Answer from the drawing. Dimensions are ordinates in mm from the lowest x, y and z of the part. Give positions to 0.01 mm unless a question says otherwise; leave off trailing zeros. Order: outer loops, then holes, each group sorted by start corner. A loop starts at its lowest first (then second) coordinate and runs counter-clockwise, first axis right, second up. Notation, with made-up numbers: M -31.75,-11 L -7.75,-11 A10 ccw -7.75,-7 Z; hole C 39,44.25 d5. An arc over 180 degrees is marked long. One line per item, written item: value.
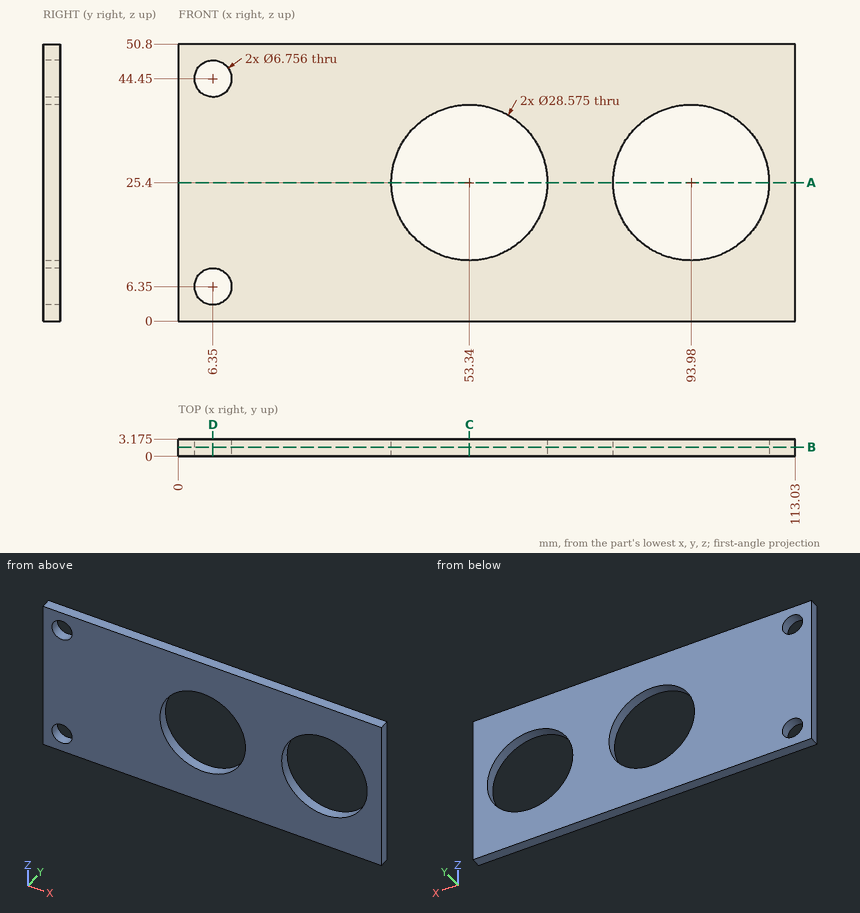
(1) Section C-C, the plane x = 53.34 is taken. Give the vertices of the cut face in (y, z) (1 decimal).
Findings:
outline: M 0,0 L 3.2,0 L 3.2,11.1 L 0,11.1 Z; M 0,39.7 L 3.2,39.7 L 3.2,50.8 L 0,50.8 Z
(2) Section A-A, the plane z = 25.4 is taken. Give the vertices of the cut face in (x, y) (1 decimal).
Findings:
outline: M 0,0 L 39.1,0 L 39.1,3.2 L 0,3.2 Z; M 67.6,0 L 79.7,0 L 79.7,3.2 L 67.6,3.2 Z; M 108.3,0 L 113,0 L 113,3.2 L 108.3,3.2 Z
(3) Section B-B, the plane y = 1.7 is taken. Give the number of separate pieces and of enclosed holes in the cut face, then the cut area to 3 significant figures.
Findings:
separate pieces: 1
enclosed holes: 4
area: 4,390 mm^2
(4) Section D-D, the plane x = 6.35 is taken. Give the vertices of the cut face in (y, z) (1 decimal), then the cut area to 3 significant figures.
Findings:
outline: M 0,0 L 3.2,0 L 3.2,3 L 0,3 Z; M 0,9.7 L 3.2,9.7 L 3.2,41.1 L 0,41.1 Z; M 0,47.8 L 3.2,47.8 L 3.2,50.8 L 0,50.8 Z
area: 118 mm^2
(5) Given P1, Ø23, axis at x = 93.98, z = 25.4, coming from the +Y side, flat-ended and moving along its own axis, determine where the tip first touches the part or whether it passes through.
Findings:
P1: passes through
(6) Find the intervals of material crossed by probe 1 along X at (y, z) = (2.75, 26) (1 decimal); probe 2 along Z at (x, y) = (53.34, 0.8); probe 3 along Z at (x, y) = (6.35, 1.45), in increasing order. Write a range as from..to.
Findings:
probe 1: x = 0..39.1, 67.6..79.7, 108.3..113
probe 2: z = 0..11.11, 39.69..50.8
probe 3: z = 0..2.97, 9.73..41.07, 47.83..50.8
